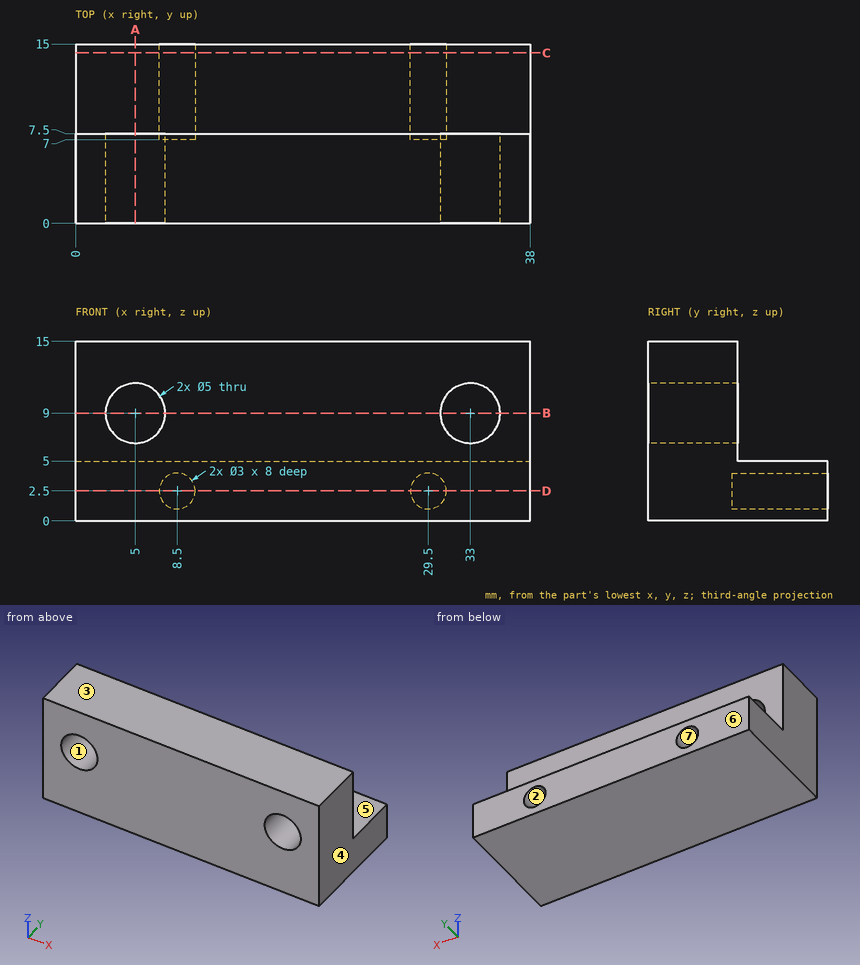
Study the drawing (mm; zero at the part's minimum x, y, z) and answer. A direction names the side the tool comes from. Coordinates: 2 decimals unless noted, no trailing zeros. Write each loop counter-clockwise with the first axis right and the second up, starting at its lowest first coordinate (ties: lowest second). Pieces come first, ordered by that corner, then holes. Notation, with made-up numbers: (-23.5, 30) - (23.5, 30) arc R22 ccw to (23.5, 43) - close; hole circle Ø6 at (17, 11.5). An arc over 180 degrees is marked (long way). Answer as a JSON object with one key per item and string values.
Q1. Find section B-B (z = 9). Write down the section's boundary in (x, y).
Results list:
{"outline": "(0, 0) - (2.5, 0) - (2.5, 7.5) - (0, 7.5) - close; (7.5, 0) - (30.5, 0) - (30.5, 7.5) - (7.5, 7.5) - close; (35.5, 0) - (38, 0) - (38, 7.5) - (35.5, 7.5) - close"}
Q2. For a pull along X with two mould halves and no side action, classify the marked faces 1, 2, 3 and 4 as pulls with the +X half, pulls with the -X half, needs draft (parallel to the pull), parting line crosses it, or undercut.
Results list:
{"face 1": "undercut", "face 2": "undercut", "face 3": "needs draft", "face 4": "pulls with the +X half"}
Q3. Find section C-C (y = 14.25). Write down the section's boundary in (x, z), plus the area to 3 significant figures.
Results list:
{"outline": "(0, 0) - (38, 0) - (38, 5) - (0, 5) - close; hole circle Ø3 at (8.5, 2.5); hole circle Ø3 at (29.5, 2.5)", "area": "176 mm^2"}
Q4. Find section D-D (z = 2.5). Write down the section's boundary in (x, y).
Results list:
{"outline": "(0, 0) - (38, 0) - (38, 15) - (31, 15) - (31, 7) - (28, 7) - (28, 15) - (10, 15) - (10, 7) - (7, 7) - (7, 15) - (0, 15) - close"}
Q5. Given pin 1 Ø4 at (x, z) = (5, 9) entering from -Y; pin 2 Ø5 at (x, z) = (24.5, 10) entering from +Y; pin 3 Ø4 at (x, y) = (11, 11) entering from +Z; pin 4 Ø1.8 at (x, z) = (29.5, 2.5) entering from +Y, each flat-ended and moving along its own axis, determine where each tip first touches the part or whether it passes through.
Results list:
{"pin 1": "passes through", "pin 2": "stops at y = 7.5", "pin 3": "stops at z = 5", "pin 4": "stops at y = 7"}
Q6. Consider L1, parallel to Z at x = 33, y = 5.75; L2, parallel to Z at x = 29.5, y = 12.5; L3, parallel to X at y = 6, z = 8.25. Determine where each line is inside the solid, lowest interval first. Write a range as from..to.
Results list:
{"L1": "z = 0..6.5, 11.5..15", "L2": "z = 0..1, 4..5", "L3": "x = 0..2.62, 7.38..30.62, 35.38..38"}
Q7. Find section A-A (x = 5). Write down the section's boundary in (y, z).
Results list:
{"outline": "(0, 0) - (15, 0) - (15, 5) - (7.5, 5) - (7.5, 6.5) - (0, 6.5) - close; (0, 11.5) - (7.5, 11.5) - (7.5, 15) - (0, 15) - close"}
Q8. Which of the six approach directions +Z, -Z, +X, -X, +Y, -Y give full straight-line access (tool end or side, diameter ignored) to the marked faces 5, 6 and 7?
Results list:
{"face 5": "+Z, +X, -X, +Y", "face 6": "+Z, -Z, +X, -X, +Y", "face 7": "+Y"}
